from build123d import *

# Parameters (mm, degrees)
CROQUIS1_W              = 68.34
CROQUIS1_H              = 81.08
SALIENTE_EXTRUIR1_DEPTH = 4
CROQUIS2_W              = 68.34
CROQUIS2_H              = 81.08
CROQUIS2_W_2            = 58.34
CROQUIS2_H_2            = 71.08
SALIENTE_EXTRUIR2_DEPTH = 17
CROQUIS3_R              = 5.5
CROQUIS3_W              = 12.087237368
CROQUIS3_H              = 5.44
CORTAR_EXTRUIR1_DEPTH   = 8
REDONDEO1_R             = 1
REDONDEO2_R             = 1


with BuildPart() as part:
    # Croquis1 → Saliente-Extruir1 (new body)
    with BuildSketch(Plane.XZ.offset(-29.575210532)):
        with Locations((26.509736299, 54.571399583)):
            Rectangle(CROQUIS1_W, CROQUIS1_H)
    extrude(amount=SALIENTE_EXTRUIR1_DEPTH)

    # Croquis2 → Saliente-Extruir2 (add)
    with BuildSketch(Plane(origin=(0, 29.575210532, 0), x_dir=(1, 0, 0), z_dir=(0, 1, 0))):
        with Locations((26.509736299, -54.571399583)):
            Rectangle(CROQUIS2_W, CROQUIS2_H)
        with Locations((26.509736299, -54.571399583)):
            Rectangle(CROQUIS2_W_2, CROQUIS2_H_2, mode=Mode.SUBTRACT)
    extrude(amount=SALIENTE_EXTRUIR2_DEPTH)

    # Croquis3 → Cortar-Extruir1 (cut)
    with BuildSketch(Plane.XY.offset(95.111399583)):
        with Locations((13.616696299, 37.550210532)):
            Circle(CROQUIS3_R)
        with Locations((43.998193346, 32.700210532)):
            Rectangle(CROQUIS3_W, CROQUIS3_H)
    extrude(amount=-CORTAR_EXTRUIR1_DEPTH, mode=Mode.SUBTRACT)

    # Redondeo1
    redondeo1_edges = [part.edges().sort_by_distance(p)[0] for p in [
        (37.954574662, 29.980210532, 92.611399583),
        (37.954574662, 35.420210532, 92.611399583),
        (50.04181203, 35.420210532, 92.611399583),
        (50.04181203, 29.980210532, 92.611399583),
    ]]
    fillet(redondeo1_edges, radius=REDONDEO1_R)

    # Redondeo2
    redondeo2_edges = [part.edges().sort_by_distance(p)[0] for p in [
        (60.679736299, 25.575210532, 54.571399583),
        (26.509736299, 46.575210532, 14.031399583),
        (-7.660263701, 46.575210532, 54.571399583),
        (26.509736299, 46.575210532, 95.111399583),
        (60.679736299, 46.575210532, 54.571399583),
        (26.509736299, 25.575210532, 95.111399583),
        (-7.660263701, 25.575210532, 54.571399583),
        (8.116696299, 37.550210532, 95.111399583),
        (37.954574662, 32.700210532, 95.111399583),
        (43.998193346, 35.420210532, 95.111399583),
        (50.04181203, 32.700210532, 95.111399583),
        (43.998193346, 29.980210532, 95.111399583),
        (38.247467881, 35.127317313, 95.111399583),
        (49.748918811, 35.127317313, 95.111399583),
        (49.748918811, 30.27310375, 95.111399583),
        (38.247467881, 30.27310375, 95.111399583),
        (-7.660263701, 36.075210532, 95.111399583),
        (60.679736299, 36.075210532, 95.111399583),
        (60.679736299, 36.075210532, 14.031399583),
        (-7.660263701, 36.075210532, 14.031399583),
        (26.509736299, 25.575210532, 14.031399583),
    ]]
    fillet(redondeo2_edges, radius=REDONDEO2_R)


solid = part.part
Geometry check sheet. Reference: the model listing, model coordinates, mm. A direction names the side the tool comes from. Coordinates: 2 decimals unless noted, no trailing zeros. Loops run counter-clockwise (first coordinate to the right, second up) from the corner with the lowest first, then second, coordinate; pieces in that order, holes last. Notation, with made-up numbers: (16.5, -34) - (30.5, -34) arc R14 cw to (30.5, -22) - close; hole circle Ø11 at (54, 86.5). An arc over 180 degrees is marked (long way). Use one line per item in the form item = value. Start each with the question number.
Item 1: Section check C-C, the plane x = 3. Enter the section's corners in (y, z).
Item 2: Gauge pin test, flat end, axial feed: pin 1 (17.5 mm diameter, centred on x = 32.5, z = 51, fed in from +Y). Record the tip position at first contact, or that the pin passes through.
Item 3: Section check B-B, the plane z = 78.5. Enter the section's corners in (x, y), and give its area (3 significant figures).
Item 4: Tool access check on faces 4 (the face through (26, 36, 95.111)), 5 (the face through (50.042, 33, 92)), 6 (the face through (26, 38, 19.031)). Record the directions out of +Z, -Z, +X, -X, +Y, -Y that give a thin tool (end or side, any length) a straight path to the whole face; none if there is none.
Item 5: Thickness scan on probe 1 along Z at (x, y) = (22, 42.25); probe 2 along X at (y, z) = (34.75, 90); probe 3 along Y at (x, z) = (52, 41.5). Record the ranges inside material, lowest first.
Item 6: Mould release check, pull along Y, two halves, no side actions. Record for faces 1 (the face through (26, 36, 14.031)), 2 (the face through (26, 25.575, 55)), 3 (the face through (44, 29.98, 92)): +Y half, -Y half, draft (parallel to the pull), parting line (faces both ways), or undercut.
Item 7: Section check A-A, the plane x = 42. Enter the section's corners in (y, z).
Computed:
q1.outline = (25.58, 15.03) arc R1 ccw to (26.58, 14.03) - (45.58, 14.03) arc R1 ccw to (46.58, 15.03) - (46.58, 19.03) - (29.58, 19.03) - (29.58, 90.11) - (46.58, 90.11) - (46.58, 94.11) arc R1 ccw to (45.58, 95.11) - (26.58, 95.11) arc R1 ccw to (25.58, 94.11) - close
q2.pin_1 = 29.58
q3.outline = (-7.66, 26.58) arc R1 ccw to (-6.66, 25.58) - (59.68, 25.58) arc R1 ccw to (60.68, 26.58) - (60.68, 45.58) arc R1 ccw to (59.68, 46.58) - (55.68, 46.58) - (55.68, 29.58) - (-2.66, 29.58) - (-2.66, 46.58) - (-6.66, 46.58) arc R1 ccw to (-7.66, 45.58) - close
q3.area = 443 mm2
q4.face_4 = +Z, +X, -X, +Y, -Y
q4.face_5 = +Z
q4.face_6 = +Y
q5.probe_1 = 14.03 to 19.03, 90.11 to 95.11
q5.probe_2 = -7.66 to -2.66, 55.68 to 60.68
q5.probe_3 = 25.58 to 29.58
q6.face_1 = draft
q6.face_2 = -Y half
q6.face_3 = undercut
q7.outline = (25.58, 15.03) arc R1 ccw to (26.58, 14.03) - (45.58, 14.03) arc R1 ccw to (46.58, 15.03) - (46.58, 19.03) - (29.58, 19.03) - (29.58, 90.11) - (29.98, 90.11) - (29.98, 94.11) arc R1 ccw to (28.98, 95.11) - (26.58, 95.11) arc R1 ccw to (25.58, 94.11) - close; (35.42, 90.11) - (46.58, 90.11) - (46.58, 94.11) arc R1 ccw to (45.58, 95.11) - (36.42, 95.11) arc R1 ccw to (35.42, 94.11) - close
